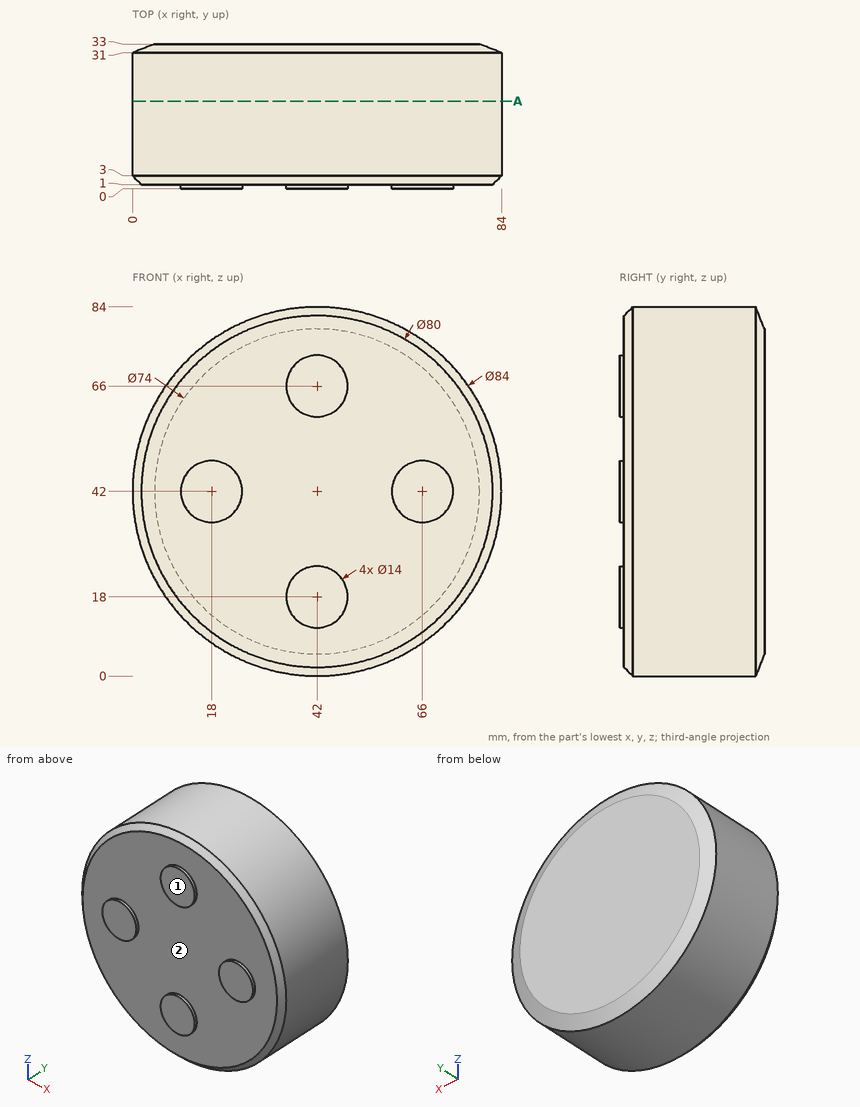
Can you work these out from the drawing? Everything is in mm from the part's minimum corner. A direction names the side the tool comes from. Give positions to 0.01 mm unless a question says otherwise; leave off trailing zeros. Order: outer loops, then holes, each group sorted by start corner. A loop starts at its lowest first (then second) coordinate and runs counter-clockwise, first axis right, second up. Notation, with made-up numbers: (52, -37.75) -> (97, -37.75) arc R11 cw to (97, -31.75) -> close; hole circle Ø9 at (-7.75, -21.75). An arc over 180 degrees is marked (long way). Return JSON: item names as keys, results as strings.
1. For pin 1 Ø8 at (x, z) = (72.5, 65.5) entering from +Y; pin 2 Ø2 at (y, z) = (29, 27.5) entering from +X; pin 3 Ø4 at (y, z) = (5, 65) entering from +X; pin 4 Ø1.5 at (y, z) = (8.5, 23) entering from +X, each with a flat end and sliding along its axis, tell me the tip position at first contact or that it passes through.
Answer list:
{"pin 1": "stops at y = 33", "pin 2": "stops at x = 81.77", "pin 3": "stops at x = 78.37", "pin 4": "stops at x = 79.83"}
2. Imagine slicing it at A-A on y = 20. List the corners of the cut face in (x, z) for me, then the cut area to 3 significant figures.
Answer list:
{"outline": "circle Ø84 at (42, 42)", "area": "5,540 mm2"}
3. On a 3-axis mill with a long thin cutter (end or side, diameter ignored), from which of +Z, -Z, +X, -X, +Y, -Y can I reach the whole of each face in a straight line? I mean the marked faces 1 and 2. Say none if no direction works.
Answer list:
{"face 1": "+Z, -Z, +X, -X, -Y", "face 2": "-Y"}
4. I need wall thicknesses on line 1 (Y direction, x = 33, z = 47); line 2 (X direction, y = 3, z = 77.5); line 3 (Y direction, x = 79.5, z = 49). Which ranges of each line are inside material? Lowest first, please. Write a range as from..to.
Answer list:
{"line 1": "y = 1..33", "line 2": "x = 19.56..64.44", "line 3": "y = 1..32.54"}
